from build123d import *

# Parameters (mm, degrees)
SKETCH1_R           = 21
BOSS_EXTRUDE1_DEPTH = 57.5
SKETCH2_R           = 2.5
BOSS_EXTRUDE2_DEPTH = 5


with BuildPart() as part:
    # Sketch1 → Boss-Extrude1 (new body)
    with BuildSketch(Plane.XY):
        Circle(SKETCH1_R)
    extrude(amount=BOSS_EXTRUDE1_DEPTH)

    # Sketch2 → Boss-Extrude2 (add)
    with BuildSketch(Plane.XY):
        with Locations((0, 14.25)):
            Circle(SKETCH2_R)
        with Locations((12.340862004, -7.125)):
            Circle(SKETCH2_R)
        with Locations((-12.340862004, -7.125)):
            Circle(SKETCH2_R)
    extrude(amount=-BOSS_EXTRUDE2_DEPTH)


solid = part.part
Part model, mm, in its own coordinate system. A direction names the side the tool comes from. Give positions to 0.01 mm unless a question says otherwise; leave off trailing zeros. Order: outer loops, then holes, each group sorted by start corner. A loop starts at its lowest first (then second) coordinate and runs counter-clockwise, first axis right, second up. Notation, with made-up numbers: (71.25, 56) -> (119.25, 56) arc R16 ccw to (119.25, 60) -> close; hole circle Ø7 at (30, -28.75). An arc over 180 degrees is marked (long way). Use one line per item in the form item = value.
(1) Pull direction X, two halves, no side cores. Call faces 1 (the face through (-12.883, -9.566, -2.465)), 2 (the face through (0, 0, 57.5)), 3 (the face through (-0.5, 11.8, -2.5)): +X half, -X half, draft (parallel to the pull), parting line (faces both ways), or undercut.
Solution:
face_1 = undercut
face_2 = draft
face_3 = parting line
(2) Saw through at C-C (z = 51.5). Write the cut outline in (x, y), then the cut area to 3 significant figures.
Solution:
outline = circle Ø42 at (0, 0)
area = 1,390 mm²
(3) Drill centre lines: line 1 (Z direction, x = -15, y = 12); line 2 (Y direction, x = 0, z = 20.5); line 3 (X direction, y = 5.5, z = 40). Where is each one in solid material? Low to high. Write a range as from..to.
Solution:
line_1 = 0..57.5
line_2 = -21..21
line_3 = -20.27..20.27
(4) Tool access for faces 4 (the face through (0, 14, -5)), 5 (the face through (0, 0, 0)): list every direction of +Z, -Z, +X, -X, +Y, -Y with a clear straight run to the whole face (end or side of a thin tool).
Solution:
face_4 = -Z, +X, -X, +Y, -Y
face_5 = -Z
(5) Saw through at B-B (y = 14.25). Write the cut outline in (x, z).
Solution:
outline = (-15.43, 0) -> (-2.5, 0) -> (-2.5, -5) -> (2.5, -5) -> (2.5, 0) -> (15.43, 0) -> (15.43, 57.5) -> (-15.43, 57.5) -> close
(6) Flat gauge pins, fed straight in: P1, Ø4, axis at y = 14, z = 36.5, coming from the +X side; P2, Ø1, axis at x = -16.5, z = 3.5, coming from the -Y side; P3, Ø5, axis at x = -5.5, y = -8.5, coming from the -Z side. Where does each tip first touch, or does it go through?
Solution:
P1 = 17.23
P2 = -13.6
P3 = 0
(7) Saw through at D-D (y = 0). Write the cut outline in (x, z).
Solution:
outline = (-21, 0) -> (21, 0) -> (21, 57.5) -> (-21, 57.5) -> close
(8) Saw through at A-A (x = 0). Write the cut outline in (y, z), then the cut area to 3 significant figures.
Solution:
outline = (-21, 0) -> (11.75, 0) -> (11.75, -5) -> (16.75, -5) -> (16.75, 0) -> (21, 0) -> (21, 57.5) -> (-21, 57.5) -> close
area = 2,440 mm²
